Design review of the part built by this model. Coordinates are the model's own, in mm. Face numbers are marked on the shaded views. A direction names the side the tool comes from. Give positions to 0.01 mm unless a question says otherwise; leave off trailing zeros. Loops run counter-clockwise (first coordinate to the right, second up) from the corner with the lowest first, then second, coordinate; pieces in that order, holes last. Notation, with made-up numbers: M 69.25,82 L 80.25,82 A30 cw 80.25,112 Z; hole C 64.25,-24.75 d8. An arc over 180 degrees is marked long. Answer as CSV lines item,"result".
```python
from build123d import *

# Parameters (mm, degrees)
F0_R     = 7.011876
F1_DEPTH = 15.24
F3_DEPTH = 7.874


with BuildPart() as f1:
    # F0 (on Front) → F1 (new body)
    with BuildSketch(Plane.XZ):
        Circle(F0_R)
    extrude(amount=F1_DEPTH)

    # F2 (on Front) → F3 (cut)
    with BuildSketch(Plane.XZ):
        Polygon((3.822133, -2.776942), (3.822133, 2.776942), (-1.459925, 4.493186), (-4.724416, 0), (-1.459925, -4.493186), align=None)
    extrude(amount=F3_DEPTH, mode=Mode.SUBTRACT)


solid = f1.part
```
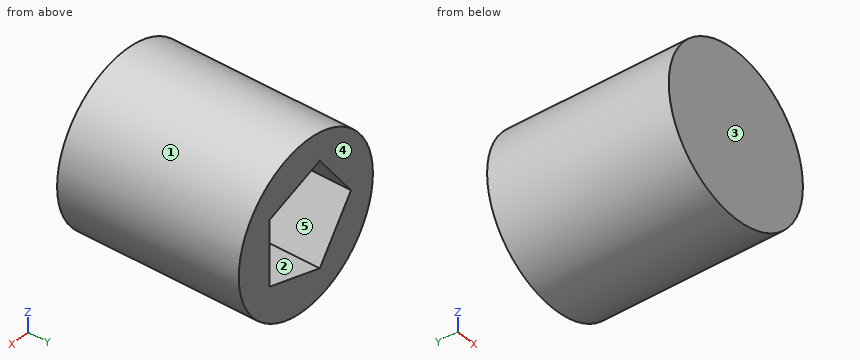
1. We need section D-D, the plane y = -8.75. Write out the cut boundary in (x, z), plus the area to 3 significant figures.
Answer block:
outline,"C 0,0 d14.02"
area,"154 mm²"
2. For the marked faces 4 and 5, list the 3-axis set-ups (+Z, -Z, +X, -X, +Y, -Y) from which the entire face can be reached by the end or side of a thin tool; tool diameter is ignored.
Answer block:
face 4,"+Z, -Z, +X, -X, +Y"
face 5,"+Y"
3. We need section A-A, the plane y = -5.25. Write out the cut boundary in (x, z), plus the area to 3 significant figures.
Answer block:
outline,"C 0,0 d14.02; hole M -4.72,0 L -1.46,-4.49 L 3.82,-2.78 L 3.82,2.78 L -1.46,4.49 Z"
area,"101 mm²"
4. To check wall thickness, follow L1, parallel to Y at x = 3.5, z = -1.75; L2, parallel to X at y = -4, z = -0.25; L3, parallel to X at y = -9, z = 0.25. State the ranges of each line that lie inside material, in increasing order. Write a range as [from, to].
Answer block:
L1,"[-15.24, -7.87]"
L2,"[-7.01, -4.54], [3.82, 7.01]"
L3,"[-7.01, 7.01]"
5. For P1, Ø2, axis at x = 4.5, y = -3, coming from the +Z side; P2, Ø1, axis at x = 5.5, z = -0.5, coming from the +Y side; P3, Ø2, axis at x = -4.5, y = -5, coming from the -Z side, all flat-tipped, find the tip position at first contact; note any pin that passes through.
Answer block:
P1,"z = 6.08"
P2,"y = 0"
P3,"z = -6.08"
6. We need section B-B, the plane z = 4. Write out the cut boundary in (x, y), plus the area to 3 significant figures.
Answer block:
outline,"M -5.76,-15.24 L 5.76,-15.24 L 5.76,0 L 0.06,0 L 0.06,-7.87 L -1.82,-7.87 L -1.82,0 L -5.76,0 Z"
area,"161 mm²"
7. The part is to be moulded in two halves that separate along X. For the marked faces 1, 2 and 3, say which applies: pulls with the +X half, pulls with the -X half, needs draft (parallel to the pull), parting line crosses it, or undercut.
Answer block:
face 1,"parting line crosses it"
face 2,"undercut"
face 3,"needs draft"
8. We need section C-C, the plane x = -0.75. Write out the cut boundary in (y, z).
Answer block:
outline,"M -15.24,-6.97 L 0,-6.97 L 0,-4.26 L -7.87,-4.26 L -7.87,4.26 L 0,4.26 L 0,6.97 L -15.24,6.97 Z"
